```python
from build123d import *

# Parameters (mm, degrees)
BASE_FLANGE1_DEPTH = 1.5875
EDGE_FLANGE1_DEPTH = 608.838


# Sheet-metal steps are written as plain solids
with BuildPart() as part:
    # Sketch1 → Base-Flange1 (new body)
    with BuildSketch(Plane(origin=(0, 0, 0), x_dir=(1, 0, 0), z_dir=(0, 1, 0))):
        Polygon((-304.419, 69.85), (-127, 69.85), (-127, 6.35), (127, 6.35), (127, 69.85), (304.419, 69.85), (304.419, -69.85), (-304.419, -69.85), align=None)
    extrude(amount=-BASE_FLANGE1_DEPTH)

    # Edge-Flange1 section (across the edge) → Edge-Flange1 (add)
    with BuildSketch(Plane(origin=(-304.419, 0, 70.5866), x_dir=(0, 0, -1), z_dir=(1, 0, 0))):
        with BuildLine():
            Line((-1.5875, 0.7366), (-1.5875, 17.4625))
            Line((-1.5875, 17.4625), (0, 17.4625))
            Line((0, 17.4625), (0, 0.7366))
            ThreePointArc((0, 0.7366), (0.215745145, 0.215745145), (0.7366, 0))
            Line((0.7366, 0), (0.7366, -1.5875))
            ThreePointArc((0.7366, -1.5875), (-0.90678687, -0.90678687), (-1.5875, 0.7366))
        make_face()
    extrude(amount=EDGE_FLANGE1_DEPTH)


solid = part.part
```
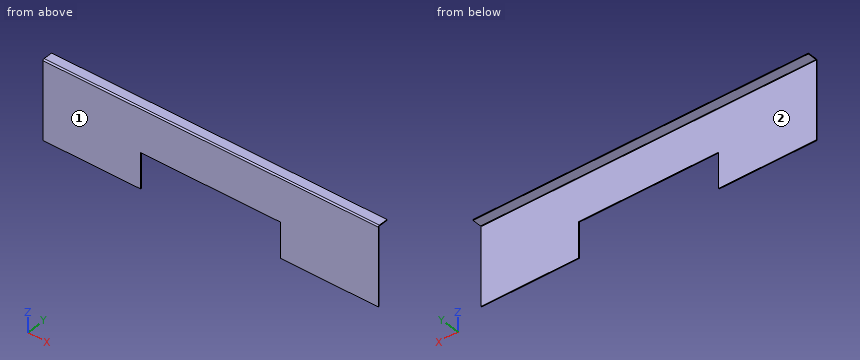
Check sheet for the modelled part. Datum: model origin and axes. Units: mm. Face numbers are marked on the shaded views. A direction names the side the tool comes from. Round coordinates to 2 decimals unless told otherwise and drop trailing zeros. Order: outer loops, then holes, each group sorted by start corner. A loop starts at its lowest first (then second) coordinate and runs counter-clockwise, first axis right, second up. Notation, with made-up numbers: M -13.5,75 L 41.5,75 A27 ccw 41.5,94 Z; hole C 41.5,55 d10. An arc over 180 degrees is marked long. Answer in a Markdown table with one row per item.
(1) Section check D-D on x = -179.5. Record the boundary of the cut face in (y, z), plus the area to 3 significant figures.
Findings:
| item | result |
|---|---|
| outline | M -1.59,-69.85 L 0,-69.85 L 0,69.85 A0.74 cw 0.74,70.59 L 17.46,70.59 L 17.46,72.17 L 0.74,72.17 A2.32 ccw -1.59,69.85 Z |
| area | 252 mm^2 |
(2) Section check C-C on y = 10.25. Record the boundary of the cut face in (x, z).
Findings:
| item | result |
|---|---|
| outline | M -304.42,70.59 L 304.42,70.59 L 304.42,72.17 L -304.42,72.17 Z |
(3) Gauge pin test, flat ends, axial feed: pin 1 (0.8 mm diameter, centred on x = -22.5, y = -0.5, fed in from -Z); pin 2 (3 mm diameter, centred on x = 111, z = -7, fed in from +Y); pin 3 (4 mm diameter, centred on x = 145.5, y = 13.5, fed in from -Z); pin 4 (3 mm diameter, centred on y = 3, z = 45, fed in from +X). Record the tip position at first contact, or that the pin passes through.
Findings:
| item | result |
|---|---|
| pin 1 | stops at z = -6.35 |
| pin 2 | stops at y = 0 |
| pin 3 | stops at z = 70.59 |
| pin 4 | passes through |
(4) Set-up check for the marked faces 1 and 2: record each of +Z, -Z, +X, -X, +Y, -Y from which the full face is reachable in a straight line by a thin tool's end or side.
Findings:
| item | result |
|---|---|
| face 1 | +Z, -Z, +X, -X, -Y |
| face 2 | -Z, +X, -X, +Y |
(5) Section check B-B on x = 22. Record the boundary of the cut face in (y, z), plus the area to 3 significant figures.
Findings:
| item | result |
|---|---|
| outline | M -1.59,-6.35 L 0,-6.35 L 0,69.85 A0.74 cw 0.74,70.59 L 17.46,70.59 L 17.46,72.17 L 0.74,72.17 A2.32 ccw -1.59,69.85 Z |
| area | 151 mm^2 |
(6) Section check A-A on z = -32.5. Record the boundary of the cut face in (x, y).
Findings:
| item | result |
|---|---|
| outline | M -304.42,-1.59 L -127,-1.59 L -127,0 L -304.42,0 Z; M 127,-1.59 L 304.42,-1.59 L 304.42,0 L 127,0 Z |
(7) Material ranges on line 1 along Y through (x, z) = (-64, 24.5); line 2 along Z through (x, y) = (-35, 11.75), recorded low to high. Write a range as from..to.
Findings:
| item | result |
|---|---|
| line 1 | y = -1.59..0 |
| line 2 | z = 70.59..72.17 |
